from build123d import *

# Parameters (mm, degrees)
EXPORT_W     = 41.596402
EXPORT_H     = 21.602024
PAD_DEPTH    = 10
EXPORT001_R  = 6.407439
PAD001_DEPTH = 1


with BuildPart() as part:
    # Export → Pad (new body)
    with BuildSketch(Plane.XY):
        with Locations((0, -0.272073)):
            Rectangle(EXPORT_W, EXPORT_H)
    extrude(amount=PAD_DEPTH)

    # Export001 (on Face6 of Pad) → Pad001 (join)
    with BuildSketch(Plane.XY.offset(10)):
        with Locations((-10.468659, 0)):
            Circle(EXPORT001_R)
        with Locations((10.468659, 0)):
            Circle(EXPORT001_R)
    extrude(amount=PAD001_DEPTH)


solid = part.part
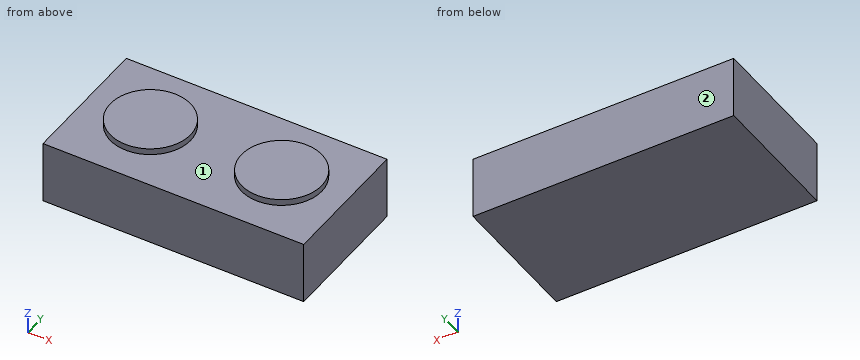
Could you check a few things on this model? Use its own coordinates, in mm. Face numbers are marked on the shaded views. A direction names the side the tool comes from. Coordinates: 2 decimals unless noted, no trailing zeros. Write each loop counter-clockwise with the first axis right and the second up, starting at its lowest first coordinate (ties: lowest second). Pieces come first, ordered by that corner, then holes. Notation, with made-up numbers: M 12,-25 L 46,-25 A15 cw 46,0 Z; hole C 86,73 d10. An arc over 180 degrees is marked long. One line per question, with ' | ' between items.
1) For the marked faces 1 and 2, which set-ups out of +Z, -Z, +X, -X, +Y, -Y let a thin tool reach every point of the face, with its end or its side?
Checks:
face 1: +Z | face 2: +Z, -Z, +X, -X, +Y
2) Imagine slicing it at C-C, the plane y = -5. Write out the boundary of the cut face in (x, z), and give its area (3 significant figures).
Checks:
outline: M -20.8,0 L 20.8,0 L 20.8,10 L 14.48,10 L 14.48,11 L 6.46,11 L 6.46,10 L -6.46,10 L -6.46,11 L -14.48,11 L -14.48,10 L -20.8,10 Z | area: 432 mm²
3) For pin 1 Ø2 at (x, y) = (-15.5, -7.5) entering from +Z; pin 2 Ø11 at (x, y) = (-4, 1.5) entering from +Z, each with a flat end and sliding along its axis, tell me the tip position at first contact or that it passes through.
Checks:
pin 1: z = 10 | pin 2: z = 11
4) Imagine slicing it at D-D, the plane y = -8. Write out the boundary of the cut face in (x, z).
Checks:
outline: M -20.8,0 L 20.8,0 L 20.8,10 L -20.8,10 Z
5) I need wall thicknesses on probe 1 along Z at (x, y) = (-17, 9.25). Which ranges of the line are inside material? Lowest first, please. Write a range as [from, to].
Checks:
probe 1: [0, 10]
6) Imagine slicing it at B-B, the plane x = -15. Write out the boundary of the cut face in (y, z).
Checks:
outline: M -11.07,0 L 10.53,0 L 10.53,10 L 4.53,10 L 4.53,11 L -4.53,11 L -4.53,10 L -11.07,10 Z
7) Imagine slicing it at A-A, the plane y = 0. Write out the boundary of the cut face in (x, z), and give its area (3 significant figures).
Checks:
outline: M -20.8,0 L 20.8,0 L 20.8,10 L 16.88,10 L 16.88,11 L 4.06,11 L 4.06,10 L -4.06,10 L -4.06,11 L -16.88,11 L -16.88,10 L -20.8,10 Z | area: 442 mm²
